from build123d import *
from build123d.topology import SkipClean

# Parameters (mm, degrees)
SKETCH1_R           = 40
BOSS_EXTRUDE1_DEPTH = 2
BOSS_EXTRUDE2_DEPTH = 6
CIRPATTERN1_COUNT   = 15
SKETCH4_R           = 1.5
CUT_EXTRUDE2_DEPTH  = 10


with BuildPart() as part:
    # Sketch1 → Boss-Extrude1 (new body)
    with BuildSketch(Plane.XY):
        Circle(SKETCH1_R)
    extrude(amount=BOSS_EXTRUDE1_DEPTH)

    # Sketch6 → Boss-Extrude2 (add)
    with SkipClean():  # the faces are left unmerged after this step: merging them gives an invalid solid
        with BuildSketch(Plane.XY):
            with BuildLine():
                Line((-1.75, 39.961700414), (-1.75, 44.961700414))
                Line((-1.75, 44.961700414), (-4.25, 44.961700414))
                Line((-4.25, 44.961700414), (-4.25, 46.961700414))
                Line((-4.25, 46.961700414), (4.25, 46.961700414))
                Line((4.25, 46.961700414), (4.25, 44.961700414))
                Line((4.25, 44.961700414), (1.75, 44.961700414))
                Line((1.75, 44.961700414), (1.75, 39.961700414))
                ThreePointArc((1.75, 39.961700414), (0, -40), (-1.75, 39.961700414))
            make_face()
        boss_extrude2 = extrude(amount=BOSS_EXTRUDE2_DEPTH)

    # CirPattern1: Boss-Extrude2 ×15 about axis
    cirpattern1_axis = Axis((0, 0, 0), (0, 0, 1))
    for i in range(1, CIRPATTERN1_COUNT):
        add(boss_extrude2.rotate(cirpattern1_axis, i * 360 / CIRPATTERN1_COUNT))

    # Sketch4 → Cut-Extrude2 (cut, symmetric)
    with BuildSketch(Plane.XY.offset(2)):
        with Locations((0, 7.5)):
            Circle(SKETCH4_R)
        with Locations((7.5, 0)):
            Circle(SKETCH4_R)
        with Locations((0, -7.5)):
            Circle(SKETCH4_R)
        with Locations((-7.5, 0)):
            Circle(SKETCH4_R)
    extrude(amount=CUT_EXTRUDE2_DEPTH, both=True, mode=Mode.SUBTRACT)


solid = part.part
Source: CAD feature listing. Evaluate the final solid. Frame: model axes, mm. A direction names the side the tool comes from. Give positions to 0.01 mm unless a question says otherwise; leave off trailing zeros. Write each loop counter-clockwise with the first axis right and the second up, starting at its lowest first coordinate (ties: lowest second). Pieces come first, ordered by that corner, then holes. Notation, with made-up numbers: (70.5, -40) -> (75.5, -40) arc R27 cw to (75.5, -10) -> close; hole circle Ø10 at (-31, -6). An arc over 180 degrees is marked (long way). Return JSON: item names as keys, results as strings. Group by question number.
1. Section C-C, the plane z = 1.4. Count the separate pieces of the cut face and the enclosed holes in it, then the cut area to 3 significant figures.
2. Section B-B, the plane y = 7.5. Output: boundary loops of the cut face in (x, z), then the cut area to 3 significant figures.
3. Mould query, pull axis X, two halves, no side actions, for faces 1 (the face through (-23.52, -35.35, 2.96)), 2 (the face through (-45, -2, 3)), 3 (the face through (-27.555, -38.028, 2.958)), 4 (the face through (27.65, -37.96, 2.96)). Classes: +X half, -X half, draft (parallel to the pull), parting line (faces both ways), or undercut.
4. Pin query (flat end, axial travel): pin 1 Ø1.8 at (x, y) = (0, -7.5) entering from -Z; pin 2 Ø1.2 at (x, z) = (-2.5, 2) entering from -Y; pin 3 Ø1 at (x, y) = (18, 18.5) entering from -Z; pin 4 Ø1.6 at (y, z) = (46, 2) entering from -X. Return the tip coordinate at first contact, or that it passes through.
5. Access query for faces 5 (the face through (-32.7, 27.09, 2.96)), 6 (the face through (46.71, -4.85, 2.96)). Directions: +Z, -Z, +X, -X, +Y, -Y. A direction counts if a zero-diameter tool reaches every point of the face in a straight line with its end or side. Return the directions, or none.
6. Material intervals for line 1 (Y direction, x = 0, z = 4.35); line 2 (Y direction, x = -26, z = 0.8); line 3 (X direction, y = 7.5, z = 4), sorted ascending. Write a range as from..to.
7. Section A-A, the plane x = 0. Output: boundary loops of the cut face in (y, z), then the cut area to 3 significant figures.
Determined:
{
 "1": {"separate pieces": "1", "enclosed holes": "4", "area": "5,510 mm2"},
 "2": {"outline": "(-39.29, 0) -> (-1.5, 0) -> (-1.5, 6) -> (-39.29, 6) -> close; (1.5, 0) -> (39.29, 0) -> (39.29, 6) -> (1.5, 6) -> close", "area": "453 mm2"},
 "3": {"face 1": "undercut", "face 2": "undercut", "face 3": "-X half", "face 4": "+X half"},
 "4": {"pin 1": "passes through", "pin 2": "stops at y = -39.95", "pin 3": "stops at z = 0", "pin 4": "stops at x = -4.25"},
 "5": {"face 5": "+Z, -Z", "face 6": "+Z, -Z, +X, -Y"},
 "6": {"line 1": "y = -40..-9, -6..6, 9..46.96", "line 2": "y = -39.16..-32.81, -30.4..30.4", "line 3": "x = -39.29..-1.5, 1.5..39.29"},
 "7": {"outline": "(-40, 0) -> (-9, 0) -> (-9, 6) -> (-40, 6) -> close; (-6, 0) -> (6, 0) -> (6, 6) -> (-6, 6) -> close; (9, 0) -> (46.96, 0) -> (46.96, 6) -> (9, 6) -> close", "area": "486 mm2"}
}
